Here's how the part is built. I have some questions about the finished solid (model axes, mm). Face numbers are marked on the shaded views. Give positions to 0.01 mm unless a question says otherwise; leave off trailing zeros. Order: outer loops, then holes, each group sorted by start corner. A loop starts at its lowest first (then second) coordinate and runs counter-clockwise, first axis right, second up. Notation, with made-up numbers: (-10, 67.5) -> (29, 67.5) arc R26 ccw to (29, 89.5) -> close; hole circle Ø7 at (-15, 84). An arc over 180 degrees is marked (long way). Write each question's results on one line, items separated by ' | '. Start each with the question number.
Q1. I'm going to push flat-ended pins straight in: pin 1 (3 mm diameter, centred on y = 11, z = -12, fed in from -X); pin 2 (2 mm diameter, centred on x = 24, y = 8.5, fed in from -Z); pin 3 (2 mm diameter, centred on x = -11, y = 7, fed in from -Z). Where does each tip first touch, or does it pass through?
Q2. I need wall thicknesses on line 1 along Z through (x, y) = (0, 16.25); line 2 along Y through (x, z) = (24, 44.5); line 3 along Y through (x, z) = (16, 14.5). Which ranges of each line are inside material? Lowest first, please. Write a range as [from, to].
Q3. Thinking about a two-plate mould opening in X: for the marked faces 1, 2 and 3, which applies, pulls with the +X half, pulls with the -X half, needs draft (parallel to the pull), parting line crosses it, or undercut?
Q4. Imagine slicing it at D-D, the plane y = 10.5. Please give me the cut outline in (x, z), then the cut area to 3 significant figures.
Q5. Imagine slicing it at A-A, the plane z = 0. Please give me the cut outline in (x, y), then the cut area to 3 significant figures.
Q6. Imagine slicing it at C-C, the plane x = 27.5. Please give me the cut outline in (y, z), then the cut area to 3 significant figures.
Q7. Imagine slicing it at B-B, the plane x = 0. Please give me the cut outline in (y, z), then the cut area to 3 significant figures.
```python
from build123d import *

# Parameters (mm, degrees)
SKETCH1_R           = 30.55
BOSS_EXTRUDE1_DEPTH = 20.32
SKETCH2_R           = 25.404
CUT_EXTRUDE1_DEPTH  = 13
SKETCH3_R           = 20
CUT_EXTRUDE2_DEPTH  = 21.32
FILLET1_R           = 1
FILLET2_R           = 1
SKETCH4_W           = 63.5
SKETCH4_H           = 101.6
SKETCH4_R           = 3.175
SKETCH4_R_2         = 26.404
BOSS_EXTRUDE2_DEPTH = 4.7625


with BuildPart() as part:
    # Sketch1 → Boss-Extrude1 (new body)
    with BuildSketch(Plane(origin=(0, 0, 0), x_dir=(1, 0, 0), z_dir=(0, 1, 0))):
        Circle(SKETCH1_R)
    extrude(amount=BOSS_EXTRUDE1_DEPTH)

    # Sketch2 → Cut-Extrude1 (cut)
    with BuildSketch(Plane.XZ):
        Circle(SKETCH2_R)
    extrude(amount=-CUT_EXTRUDE1_DEPTH, mode=Mode.SUBTRACT)

    # Sketch3 → Cut-Extrude2 (cut, through all)
    with BuildSketch(Plane(origin=(0, 20.32, 0), x_dir=(1, 0, 0), z_dir=(0, 1, 0))):
        Circle(SKETCH3_R)
    extrude(amount=-CUT_EXTRUDE2_DEPTH, mode=Mode.SUBTRACT)

    # Fillet1
    fillet1_edges = [part.edges().sort_by_distance(p)[0] for p in [
        (-25.404, 0, 0),
    ]]
    fillet(fillet1_edges, radius=FILLET1_R)

    # Fillet2
    fillet2_edges = [part.edges().sort_by_distance(p)[0] for p in [
        (-20, 13, 0),
    ]]
    fillet(fillet2_edges, radius=FILLET2_R)

    # Sketch4 → Boss-Extrude2 (add)
    with BuildSketch(Plane.XZ):
        Rectangle(SKETCH4_W, SKETCH4_H)
        with Locations((-22.225, 41.275)):
            Circle(SKETCH4_R, mode=Mode.SUBTRACT)
        with Locations((22.225, 41.275)):
            Circle(SKETCH4_R, mode=Mode.SUBTRACT)
        with Locations((22.225, -41.275)):
            Circle(SKETCH4_R, mode=Mode.SUBTRACT)
        with Locations((-22.225, -41.275)):
            Circle(SKETCH4_R, mode=Mode.SUBTRACT)
        Circle(SKETCH4_R_2, mode=Mode.SUBTRACT)
    extrude(amount=-BOSS_EXTRUDE2_DEPTH)


solid = part.part
```
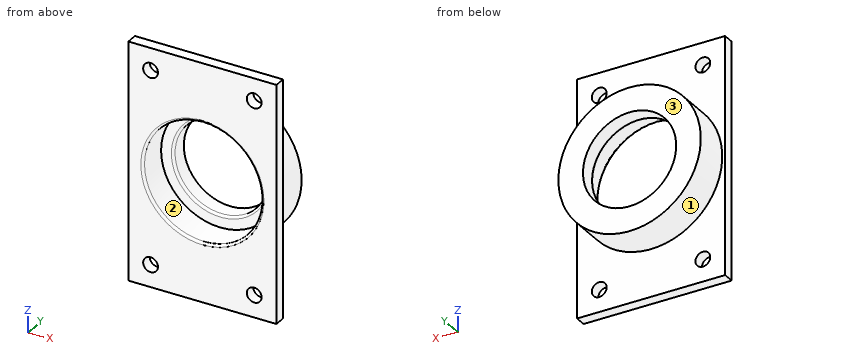
Geometry check:
1) pin 1: x = -28.69 | pin 2: z = -20.11 | pin 3: z = -28.87
2) line 1: [-30.55, -20], [20, 30.55] | line 2: [0, 4.76] | line 3: [13, 20.32]
3) face 1: parting line crosses it | face 2: undercut | face 3: needs draft
4) outline: circle Ø61.1 at (0, 0); hole circle Ø50.81 at (0, 0) | area: 905 mm²
5) outline: (-31.75, 0) -> (-26.4, 0) arc R1 ccw to (-25.4, 1) -> (-25.4, 13) -> (-21, 13) arc R1 ccw to (-20, 14) -> (-20, 20.32) -> (-30.55, 20.32) -> (-30.55, 4.76) -> (-31.75, 4.76) -> close; (20, 14) arc R1 ccw to (21, 13) -> (25.4, 13) -> (25.4, 1) arc R1 ccw to (26.4, 0) -> (31.75, 0) -> (31.75, 4.76) -> (30.55, 4.76) -> (30.55, 20.32) -> (20, 20.32) -> close | area: 299 mm²
6) outline: (0, -50.8) -> (4.76, -50.8) -> (4.76, -13.31) -> (20.32, -13.31) -> (20.32, 13.31) -> (4.76, 13.31) -> (4.76, 50.8) -> (0, 50.8) -> close | area: 898 mm²
7) outline: (0, -50.8) -> (4.76, -50.8) -> (4.76, -30.55) -> (20.32, -30.55) -> (20.32, -20) -> (14, -20) arc R1 ccw to (13, -21) -> (13, -25.4) -> (1, -25.4) arc R1 ccw to (0, -26.4) -> close; (0, 26.4) arc R1 ccw to (1, 25.4) -> (13, 25.4) -> (13, 21) arc R1 ccw to (14, 20) -> (20.32, 20) -> (20.32, 30.55) -> (4.76, 30.55) -> (4.76, 50.8) -> (0, 50.8) -> close | area: 480 mm²
